```python
from build123d import *

# Parameters (mm, degrees)
SKETCH_1_W          = 20
SKETCH_1_H          = 20
EXTRUDE_1_DEPTH     = 40
SKETCH_2_W          = 17
SKETCH_2_H          = 17
EXTRUDE_2_DEPTH     = 10
SKETCH_3_W          = 15
SKETCH_3_H          = 15
EXTRUDE_3_DEPTH     = 5
SKETCH_4_R          = 3.745
CUT_EXTRUDE_1_DEPTH = 2


with BuildPart() as part:
    # ｽｹｯﾁ1 → ﾎﾞｽ - 押し出し1 (new body)
    with BuildSketch(Plane.XY):
        Rectangle(SKETCH_1_W, SKETCH_1_H)
    extrude(amount=EXTRUDE_1_DEPTH)

    # ｽｹｯﾁ2 → ﾎﾞｽ - 押し出し2 (add)
    with BuildSketch(Plane.XY.offset(40)):
        Rectangle(SKETCH_2_W, SKETCH_2_H)
    extrude(amount=EXTRUDE_2_DEPTH)

    # ｽｹｯﾁ3 → ﾎﾞｽ - 押し出し3 (add)
    with BuildSketch(Plane.XY.offset(50)):
        Rectangle(SKETCH_3_W, SKETCH_3_H)
    extrude(amount=EXTRUDE_3_DEPTH)

    # ｽｹｯﾁ4 → ｶｯﾄ - 押し出し1 (cut)
    with BuildSketch(Plane.XY.offset(55)):
        with Locations((-3.75, 3.75)):
            Circle(SKETCH_4_R)
        with Locations(Location((3.75, 3.75, 0), (0, 0, 180))):
            Circle(SKETCH_4_R)
        with Locations((3.75, -3.75)):
            Circle(SKETCH_4_R)
        with Locations(Location((-3.75, -3.75, 0), (0, 0, 180))):
            Circle(SKETCH_4_R)
    extrude(amount=-CUT_EXTRUDE_1_DEPTH, mode=Mode.SUBTRACT)


solid = part.part
```
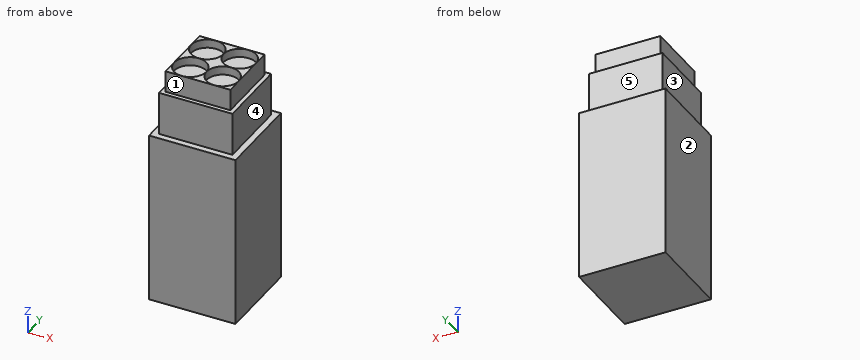
Work out the finished part from the listing and answer in its coordinate system (mm). Face numbers are marked on the shaded views. A direction names the side the tool comes from. Round coordinates to 2 decimals unless told otherwise and drop trailing zeros. Loops run counter-clockwise (first coordinate to the right, second up) from the corner with the lowest first, then second, coordinate; pieces in that order, holes last. Notation, with made-up numbers: M 7.25,-22 L 28.25,-22 A28 cw 28.25,4 Z; hole C 71,-21 d2. An arc over 180 degrees is marked long. One line per question, with ' | ' between items.
Q1. Find section C-C, the plane z = 48.5. Give the vertices of the cut face in (x, y).
Conclusion:
outline: M -8.5,-8.5 L 8.5,-8.5 L 8.5,8.5 L -8.5,8.5 Z
Q2. Find section A-A, the plane y = -3.75. Give the vertices of the cut face in (x, z) (3 decimals).
Conclusion:
outline: M -10,0 L 10,0 L 10,40 L 8.5,40 L 8.5,50 L 7.5,50 L 7.5,55 L 7.495,55 L 7.495,53 L 0.005,53 L 0.005,55 L -0.005,55 L -0.005,53 L -7.495,53 L -7.495,55 L -7.5,55 L -7.5,50 L -8.5,50 L -8.5,40 L -10,40 Z
Q3. Each of these flat-tipped pins is pushed along its axis until it touches: pin 1 Ø5 at (x, z) = (1, 43.5) entering from +Y; pin 2 Ø5 at (y, z) = (-3.5, 46) entering from -X; pin 3 Ø3.5 at (x, y) = (-4, 2.5) entering from +Z. Where does it stop, or does it pass through?
Conclusion:
pin 1: stops at y = 8.5 | pin 2: stops at x = -8.5 | pin 3: stops at z = 53
Q4. A tool of negligible diameter and unlimited length cuts with its end or side. For the marked faces 1, 2, 3, 4 and 5, from which of +Z, -Z, +X, -X, +Y, -Y can it reach the whole face along a straight path? Write none if from no direction.
Conclusion:
face 1: +Z, +X, -X, -Y | face 2: +Z, -Z, -X, +Y, -Y | face 3: +Z, -X, +Y, -Y | face 4: +Z, +X, +Y, -Y | face 5: +Z, +X, -X, +Y
Q5. Consider line 1 along Z through (x, y) = (9.25, -8); line 2 along Z through (x, y) = (-2.75, -6.25); line 3 along Y through (x, z) = (1, 47.5). Determine where each line is inside the solid, lowest interval first. Write a range as from..to.
Conclusion:
line 1: z = 0..40 | line 2: z = 0..53 | line 3: y = -8.5..8.5
